```python
from build123d import *

# Parameters (mm, degrees)
F0_W     = 63.5
F0_H     = 76.2
F1_DEPTH = 101.6
F3_DEPTH = 144.018
F4_W     = 12.4857110355
F4_H     = 50.8
F4_W_2   = 12.9142889645
F5_DEPTH = 38.1


with BuildPart() as f1:
    # F0 (on Front) → F1 (new body)
    with BuildSketch(Plane.XZ):
        with Locations((-20.1713825464, 1.844201237)):
            Rectangle(F0_W, F0_H)
    extrude(amount=F1_DEPTH)

    # F2 (on face) → F3 (cut)
    with BuildSketch(Plane.XZ.offset(101.6)):
        with BuildLine():
            ThreePointArc((11.5786174536, -10.632746352), (32.6080102155, 4.0376145015), (40.6873602154, 28.372341767))
            ThreePointArc((40.6873602154, 28.372341767), (5.8466064421, 68.6374442058), (-39.0070935819, 39.944201237))
            Line((-39.0070935819, 39.944201237), (11.5786174536, 39.944201237))
            Line((11.5786174536, 39.944201237), (11.5786174536, -10.632746352))
        make_face()
        with BuildLine():
            Line((11.5786174536, 39.944201237), (-39.0070935819, 39.944201237))
            ThreePointArc((-39.0070935819, 39.944201237), (-28.7678159153, -0.4004587357), (11.5786174536, -10.632746352))
            Line((11.5786174536, -10.632746352), (11.5786174536, 39.944201237))
        make_face()
    extrude(amount=-F3_DEPTH, mode=Mode.SUBTRACT)

    # F4 (on face) → F5 (cut)
    with BuildSketch(Plane.XY.offset(39.944201237)):
        with Locations((-32.7642380642, -50.8)):
            Rectangle(F4_W, F4_H)
        with Locations((-45.4642380642, -50.8)):
            Rectangle(F4_W_2, F4_H)
    extrude(amount=-F5_DEPTH, mode=Mode.SUBTRACT)


solid = f1.part
```
Geometry check sheet. Reference: the model listing, model coordinates, mm. A direction names the side the tool comes from. Round coordinates to 2 decimals unless told otherwise and drop trailing zeros. Loops run counter-clockwise (first coordinate to the right, second up) from the corner with the lowest first, then second, coordinate; pieces in that order, holes last. Notation, with made-up numbers: (19.25, 6.5) - (69.25, 6.5) arc R19 cw to (69.25, 11.5) - close; hole circle Ø10 at (8.25, 65). An arc over 180 degrees is marked (long way). Write item = value, one per line. Start each with the question number.
1. Mould release check, pull along Y, two halves, no side actions. Record for faces 3 (the face through (-42, -50, 1.844)), 4 (the face through (-28, 0, -15)), 5 (the face through (-46, -13, 39.944)): released by +Y, released by -Y, zero draft, split by the parting line, or undercut.
2. Set-up check for faces 1 (the face through (11.579, -50, -24)), 2 (the face through (-46, -76.2, 21)): record each of +Z, -Z, +X, -X, +Y, -Y from which the full face is reachable in a straight line by a thin tool's end or side.
3. Thickness scan on line 1 (Z direction, x = -1, y = -33); line 2 (Z direction, x = -24, y = -65.5); line 3 (X direction, y = -38, z = -7.5). Record the ranges inside material, lowest first.
4. Section check B-B on x = -45. Enter the section's corners in (y, z).
5. Section check A-A on z = 9.5. Enter the section's corners in (x, y).
6. Depth check by flat-ended pin: pin 1 (12 mm diameter, centred on y = -16.5, z = 31, fed in from +X); pin 2 (3 mm diameter, centred on x = -22.5, y = -12.5, fed in from +Z); pin 3 (17 mm diameter, centred on x = -44.5, y = -50, fed in from +Z). Enter the tip coordinate at first touch or a pass-through.
7. Section check D-D on z = 19. Enter the section's corners in (x, y), then the cut area to 3 significant figures.
8. Section check C-C on y = -47.5. Enter the section's corners in (x, z), then the cut area to 3 significant figures.
Working result:
q1.face_3 = undercut
q1.face_4 = released by +Y
q1.face_5 = zero draft
q2.face_1 = +Z, -Z, +X, +Y, -Y
q2.face_2 = +Z, +X, -X
q3.line_1 = -36.26 to -12.3
q3.line_2 = -36.26 to -4.48
q3.line_3 = -51.92 to -19.2
q4.outline = (-101.6, -36.26) - (0, -36.26) - (0, 39.94) - (-25.4, 39.94) - (-25.4, 1.84) - (-76.2, 1.84) - (-76.2, 39.94) - (-101.6, 39.94) - close
q5.outline = (-51.92, -101.6) - (-36.05, -101.6) - (-36.05, -76.2) - (-51.92, -76.2) - close; (-51.92, -25.4) - (-36.05, -25.4) - (-36.05, 0) - (-51.92, 0) - close
q6.pin_1 = -39.76
q6.pin_2 = -4.48
q6.pin_3 = 1.84
q7.outline = (-51.92, -101.6) - (-39.59, -101.6) - (-39.59, -76.2) - (-51.92, -76.2) - close; (-51.92, -25.4) - (-39.59, -25.4) - (-39.59, 0) - (-51.92, 0) - close
q7.area = 626 mm^2
q8.outline = (-51.92, -36.26) - (11.58, -36.26) - (11.58, -10.63) arc R40.69 cw to (-30.85, 1.84) - (-51.92, 1.84) - close
q8.area = 1,960 mm^2
